Input: part model. Units: mm. Frame: model coordinates. A direction names the side the tool comes from. Give positions to 0.01 mm unless a question says otherwise; leave off trailing zeros. Loops run counter-clockwise (first coordinate to the right, second up) from the corner with the lowest first, then second, coordinate; pieces in that order, holes last. Notation, with made-up numbers: M 11,-24 L 44,-24 A9 cw 44,-19 Z; hole C 55.5,8.5 d5. An arc over 180 degrees is marked long. Answer as a JSON object with one key per item and string values. Group by question number.
```python
from build123d import *

# Parameters (mm, degrees)
SKETCH1_R           = 100
BOSS_EXTRUDE1_DEPTH = 100
SKETCH2_R           = 90
CUT_EXTRUDE1_DEPTH  = 90
FILLET1_R           = 10
SKETCH3_R           = 5
BOSS_EXTRUDE2_DEPTH = 5
SKETCH4_R           = 3
CUT_EXTRUDE2_DEPTH  = 5


with BuildPart() as part:
    # Sketch1 → Boss-Extrude1 (new body)
    with BuildSketch(Plane(origin=(0, 0, 0), x_dir=(1, 0, 0), z_dir=(0, 1, 0))):
        with Locations(Location((0, 0, 0), (0, 0, 270))):
            Circle(SKETCH1_R)
    extrude(amount=BOSS_EXTRUDE1_DEPTH)

    # Sketch2 → Cut-Extrude1 (cut)
    with BuildSketch(Plane(origin=(0, 100, 0), x_dir=(1, 0, 0), z_dir=(0, 1, 0))):
        with Locations(Location((0, 0, 0), (0, 0, 270))):
            Circle(SKETCH2_R)
    extrude(amount=-CUT_EXTRUDE1_DEPTH, mode=Mode.SUBTRACT)

    # Fillet1
    fillet1_edges = [part.edges().sort_by_distance(p)[0] for p in [
        (0, 0, -100),
    ]]
    fillet(fillet1_edges, radius=FILLET1_R)

    # Sketch3 → Boss-Extrude2 (add)
    with BuildSketch(Plane.XZ):
        with Locations(Location((0, 0, 0), (0, 0, 90))):
            Circle(SKETCH3_R)
    extrude(amount=BOSS_EXTRUDE2_DEPTH)

    # Sketch4 → Cut-Extrude2 (cut)
    with BuildSketch(Plane(origin=(0, -5, 0), x_dir=(-1, 0, 0), z_dir=(0, -1, 0))):
        with Locations(Location((0, 0, 0), (0, 0, 90))):
            Circle(SKETCH4_R)
    extrude(amount=-CUT_EXTRUDE2_DEPTH, mode=Mode.SUBTRACT)


solid = part.part
```
1. Reachability of faces 1 (the flat face through (38, 100, -82)), 2 (the flat face through (1, 10, -1)), 3 (the flat face through (0, 0, 0)) from +Z, -Z, +X, -X, +Y, -Y: full face, straight path, thin tool, end or side. Return the list, or none.
2. First-contact query: P1, Ø1.5, axis at x = -2, y = 44, coming from the +Z side; P2, Ø4, axis at x = -24.5, y = 15.5, coming from the +Z side; P3, Ø4, axis at x = 77.5, z = 53.5, coming from the -Y side. Flat tips, straight axial feed; report the tip coordinate or a pass-through.
3. Mould query, pull axis X, two halves, no side actions, for faces 4 (the cylindrical face through (4.88, -2.46, -1.08)), 5 (the flat face through (3.3, -5, -0.1)), 6 (the cylindrical face through (-34.471, 55.63, 83.137)). Classes: pulls with the +X half, pulls with the -X half, needs draft (parallel to the pull), parting line crosses it, or undercut.
4. Section A-A (x = 0). Output: boundary loops of the cut face in (y, z), then the cut area to 3 significant figures.
5. Section C-C (y = 51.5). Output: boundary loops of the cut face in (x, z).
6. Section B-B (z = 0). Output: boundary loops of the cut face in (x, y), then the cut area to 3 significant figures.
7. Material intervals for L1, parallel to X at y = -2.55, z = 0; L2, parallel to X at y = 29.5, z = 0; L3, parallel to Y at x = -43, z = 6.5, sorted ascending.
Geometry results:
{
 "1": {"face 1": "+Z, -Z, +X, -X, +Y", "face 2": "+Y", "face 3": "-Y"},
 "2": {"P1": "z = 99.99", "P2": "z = 97.44", "P3": "y = 0.24"},
 "3": {"face 4": "parting line crosses it", "face 5": "needs draft", "face 6": "undercut"},
 "4": {"outline": "M -5,-5 L 0,-5 L 0,-90 A10 ccw 10,-100 L 100,-100 L 100,-90 L 10,-90 L 10,90 L 100,90 L 100,100 L 10,100 A10 ccw 0,90 L 0,5 L -5,5 L -5,3 L 0,3 L 0,-3 L -5,-3 Z", "area": "3,780 mm2"},
 "5": {"outline": "C 0,0 d200; hole C 0,0 d180"},
 "6": {"outline": "M -100,10 A10 ccw -90,0 L -5,0 L -5,-5 L -3,-5 L -3,0 L 3,0 L 3,-5 L 5,-5 L 5,0 L 90,0 A10 ccw 100,10 L 100,100 L 90,100 L 90,10 L -90,10 L -90,100 L -100,100 Z", "area": "3,780 mm2"},
 "7": {"L1": "-5 to -3, 3 to 5", "L2": "-100 to -90, 90 to 100", "L3": "0 to 10"}
}
